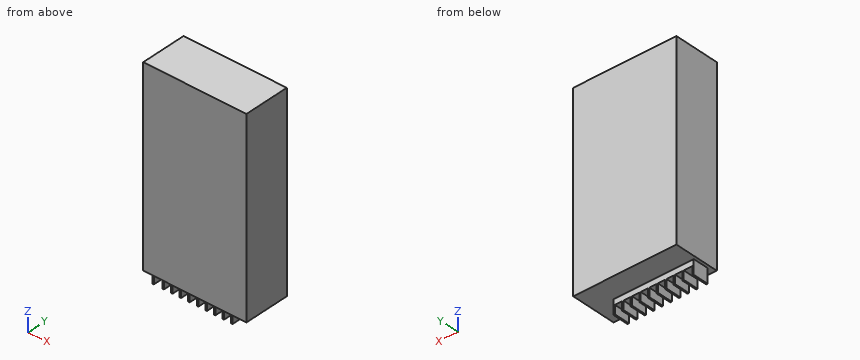
Autodesk Inventor part; units mm, degrees
ref_plane "YZ Plane" through (0, 0, 0) normal (1, 0, 0) x (0, 1, 0)
ref_plane "XZ Plane" through (0, 0, 0) normal (0, 1, 0) x (-1, 0, 0)
ref_plane "XY Plane" through (0, 0, 0) normal (0, 0, 1) x (1, 0, 0)
sketch "Sketch1" plane through (0, 0, 0) normal (0, 0, 1) x (1, 0, 0)
  line L0 (0, 0) -> (114.3, 0)
  line L1 (114.3, 0) -> (114.3, 50.8)
  line L2 (114.3, 50.8) -> (0, 50.8)
  line L3 (0, 50.8) -> (0, 0)
  dimension "d0" = 114.3
  dimension "d1" = 50.8
extrude "Extrusion1" add sketch "Sketch1" against normal blind 211.1375
sketch "Sketch2" plane through (0, 0, -211.1375) normal (0, 0, -1) x (-1, 0, 0)
  line L0 (-114.3, 0) -> (0, 0)
  line L1 (0, 0) -> (0, 50.8)
  line L2 (0, 50.8) -> (-114.3, 50.8)
  line L3 (-114.3, 50.8) -> (-114.3, 0)
  line L4 (-3.175, 7.9375) -> (-92.075, 7.9375)
  line L5 (-92.075, 7.9375) -> (-92.075, 25.4)
  line L6 (-92.075, 25.4) -> (-3.175, 25.4)
  line L7 (-3.175, 25.4) -> (-3.175, 7.9375)
  line L8 (-82.55, 25.4) -> (-80.9625, 25.4)
  line L9 (-80.9625, 25.4) -> (-80.9625, 7.9375)
  line L10 (-80.9625, 7.9375) -> (-82.55, 7.9375)
  line L11 (-82.55, 7.9375) -> (-82.55, 25.4)
  line L12 (-73.025, 25.4) -> (-71.4375, 25.4)
  line L13 (-71.4375, 25.4) -> (-71.4375, 7.9375)
  line L14 (-71.4375, 7.9375) -> (-73.025, 7.9375)
  line L15 (-73.025, 7.9375) -> (-73.025, 25.4)
  line L16 (-63.5, 25.4) -> (-61.9125, 25.4)
  line L17 (-61.9125, 25.4) -> (-61.9125, 7.9375)
  line L18 (-61.9125, 7.9375) -> (-63.5, 7.9375)
  line L19 (-63.5, 7.9375) -> (-63.5, 25.4)
  line L20 (-53.975, 25.4) -> (-52.3875, 25.4)
  line L21 (-52.3875, 25.4) -> (-52.3875, 7.9375)
  line L22 (-52.3875, 7.9375) -> (-53.975, 7.9375)
  line L23 (-53.975, 7.9375) -> (-53.975, 25.4)
  line L24 (-44.45, 25.4) -> (-42.8625, 25.4)
  line L25 (-42.8625, 25.4) -> (-42.8625, 7.9375)
  line L26 (-42.8625, 7.9375) -> (-44.45, 7.9375)
  line L27 (-44.45, 7.9375) -> (-44.45, 25.4)
  line L28 (-34.925, 25.4) -> (-33.3375, 25.4)
  line L29 (-33.3375, 25.4) -> (-33.3375, 7.9375)
  line L30 (-33.3375, 7.9375) -> (-34.925, 7.9375)
  line L31 (-34.925, 7.9375) -> (-34.925, 25.4)
  line L32 (-25.4, 25.4) -> (-23.8125, 25.4)
  line L33 (-23.8125, 25.4) -> (-23.8125, 7.9375)
  line L34 (-23.8125, 7.9375) -> (-25.4, 7.9375)
  line L35 (-25.4, 7.9375) -> (-25.4, 25.4)
  line L36 (-15.875, 25.4) -> (-14.2875, 25.4)
  line L37 (-14.2875, 25.4) -> (-14.2875, 7.9375)
  line L38 (-14.2875, 7.9375) -> (-15.875, 7.9375)
  line L39 (-15.875, 7.9375) -> (-15.875, 25.4)
  line L40 (-4.7625, 25.4) -> (-3.175, 25.4)
  line L41 (-3.175, 25.4) -> (-3.175, 7.9375)
  line L42 (-3.175, 7.9375) -> (-4.7625, 7.9375)
  line L43 (-4.7625, 7.9375) -> (-4.7625, 25.4)
  line L44 (-90.4875, 25.4) -> (-92.075, 25.4)
  line L45 (-92.075, 25.4) -> (-92.075, 7.9375)
  line L46 (-92.075, 7.9375) -> (-90.4875, 7.9375)
  line L47 (-90.4875, 7.9375) -> (-90.4875, 25.4)
  dimension "d4" = 3.175
  dimension "d5" = 7.9375
  dimension "d6" = 22.225
  dimension "d7" = 25.4
  dimension "d8" = 1.5875
  dimension "d9" = 7.9375
  dimension "d10" = 1.5875
  dimension "d11" = 7.9375
  dimension "d12" = 1.5875
  dimension "d13" = 7.9375
  dimension "d14" = 1.5875
  dimension "d15" = 7.9375
  dimension "d16" = 1.5875
  dimension "d17" = 7.9375
  dimension "d18" = 1.5875
  dimension "d19" = 1.5875
  dimension "d21" = 1.5875
  dimension "d23" = 1.5875
  dimension "d24" = 7.9375
  dimension "d25" = 1.5875
  dimension "d26" = 7.9375
  dimension "d27" = 7.9375
extrude "Extrusion2" add sketch "Sketch2" along normal blind 15.875 contours L4 L43 L6 L7 | L4 L39 L6 L37 | L4 L35 L6 L33 | L4 L31 L6 L29 | L4 L27 L6 L25 | L4 L23 L6 L21 | L4 L19 L6 L17 | L4 L15 L6 L13 | L4 L11 L6 L9 | L4 L5 L6 L47
sketch "Sketch3" plane through (0, 0, -211.1375) normal (0, 0, -1) x (-1, 0, 0)
  line L0 (-71.4375, 7.9375) -> (-73.025, 7.9375)
  line L1 (-73.025, 7.9375) -> (-73.025, 25.4)
  line L2 (-52.3875, 7.9375) -> (-53.975, 7.9375)
  line L3 (-53.975, 7.9375) -> (-53.975, 25.4)
  line L4 (-33.3375, 7.9375) -> (-34.925, 7.9375)
  line L5 (-34.925, 7.9375) -> (-34.925, 25.4)
  line L6 (-23.8125, 7.9375) -> (-25.4, 7.9375)
  line L7 (-25.4, 7.9375) -> (-25.4, 25.4)
  line L8 (-14.2875, 7.9375) -> (-15.875, 7.9375)
  line L9 (-15.875, 7.9375) -> (-15.875, 25.4)
  line L10 (-42.8625, 7.9375) -> (-44.45, 7.9375)
  line L11 (-44.45, 7.9375) -> (-44.45, 25.4)
  line L12 (-61.9125, 7.9375) -> (-63.5, 7.9375)
  line L13 (-63.5, 7.9375) -> (-63.5, 25.4)
  line L14 (-80.9625, 7.9375) -> (-82.55, 7.9375)
  line L15 (-82.55, 7.9375) -> (-82.55, 25.4)
  line L16 (-92.075, 25.4) -> (-3.175, 25.4)
  line L17 (-3.175, 25.4) -> (-3.175, 7.9375)
  line L18 (-3.175, 7.9375) -> (-92.075, 7.9375)
  line L19 (-92.075, 7.9375) -> (-92.075, 25.4)
  line L20 (-90.4875, 7.9375) -> (-92.075, 7.9375)
  line L21 (-92.075, 7.9375) -> (-92.075, 25.4)
  line L22 (-92.075, 25.4) -> (-90.4875, 25.4)
  line L23 (-90.4875, 25.4) -> (-90.4875, 7.9375)
  line L24 (-82.55, 25.4) -> (-80.9625, 25.4)
  line L25 (-80.9625, 25.4) -> (-80.9625, 7.9375)
  line L26 (-80.9625, 7.9375) -> (-82.55, 7.9375)
  line L27 (-82.55, 7.9375) -> (-82.55, 25.4)
  line L28 (-73.025, 25.4) -> (-71.4375, 25.4)
  line L29 (-71.4375, 25.4) -> (-71.4375, 7.9375)
  line L30 (-71.4375, 7.9375) -> (-73.025, 7.9375)
  line L31 (-73.025, 7.9375) -> (-73.025, 25.4)
  line L32 (-63.5, 25.4) -> (-61.9125, 25.4)
  line L33 (-61.9125, 25.4) -> (-61.9125, 7.9375)
  line L34 (-61.9125, 7.9375) -> (-63.5, 7.9375)
  line L35 (-63.5, 7.9375) -> (-63.5, 25.4)
  line L36 (-53.975, 25.4) -> (-52.3875, 25.4)
  line L37 (-52.3875, 25.4) -> (-52.3875, 7.9375)
  line L38 (-52.3875, 7.9375) -> (-53.975, 7.9375)
  line L39 (-53.975, 7.9375) -> (-53.975, 25.4)
  line L40 (-44.45, 25.4) -> (-42.8625, 25.4)
  line L41 (-42.8625, 25.4) -> (-42.8625, 7.9375)
  line L42 (-42.8625, 7.9375) -> (-44.45, 7.9375)
  line L43 (-44.45, 7.9375) -> (-44.45, 25.4)
  line L44 (-34.925, 25.4) -> (-33.3375, 25.4)
  line L45 (-33.3375, 25.4) -> (-33.3375, 7.9375)
  line L46 (-33.3375, 7.9375) -> (-34.925, 7.9375)
  line L47 (-34.925, 7.9375) -> (-34.925, 25.4)
  line L48 (-25.4, 25.4) -> (-23.8125, 25.4)
  line L49 (-23.8125, 25.4) -> (-23.8125, 7.9375)
  line L50 (-23.8125, 7.9375) -> (-25.4, 7.9375)
  line L51 (-25.4, 7.9375) -> (-25.4, 25.4)
  line L52 (-15.875, 25.4) -> (-14.2875, 25.4)
  line L53 (-14.2875, 25.4) -> (-14.2875, 7.9375)
  line L54 (-14.2875, 7.9375) -> (-15.875, 7.9375)
  line L55 (-15.875, 7.9375) -> (-15.875, 25.4)
  line L56 (-4.7625, 25.4) -> (-3.175, 25.4)
  line L57 (-3.175, 25.4) -> (-3.175, 7.9375)
  line L58 (-3.175, 7.9375) -> (-4.7625, 7.9375)
  line L59 (-4.7625, 7.9375) -> (-4.7625, 25.4)
extrude "Extrusion3" add sketch "Sketch3" along normal blind 6.35 contours L29 L16 L13 L18 | L18 L25 L16 L1 | L33 L16 L3 L18 | L18 L23 L16 L15 | L37 L16 L11 L18 | L41 L16 L5 L18 | L45 L16 L7 L18 | L49 L16 L9 L18 | L53 L16 L59 L18
properties part number "powerSupply"
Input: part model. Units: mm. Frame: model coordinates. Give positions to 0.01 mm unless a question says otherwise; leave off trailing zeros. Write each loop counter-clockwise with the first axis right and the second up, starting at its lowest first coordinate (ties: lowest second). Pieces come first, ordered by that corner, then holes. Notation, with made-up numbers: M 45,83 L 69,83 A12 cw 69,105 Z; hole C 57.5,68.25 d10. An arc over 180 degrees is marked long. Use one line per item in the form item = value.
1. Cut plane B-B on y = 5.5. Return loops of the section in (x, z), and give its area (3 significant figures).
Outcome:
outline = M 0,-211.14 L 114.3,-211.14 L 114.3,0 L 0,0 Z
area = 24,100 mm²
2. Cut plane A-A on x = 47.5. Return loops of the section in (y, z).
Outcome:
outline = M 0,-211.14 L 7.94,-211.14 L 7.94,-217.49 L 25.4,-217.49 L 25.4,-211.14 L 50.8,-211.14 L 50.8,0 L 0,0 Z
3. Ray query, L1, parallel to Z at x = 82.5, y = 45; L2, parallel to Z at x = 67, y = 21.5. Return the intervals inside material, ascending.
Outcome:
L1 = -211.14 to 0
L2 = -217.49 to 0
4. Cut plane C-C on x = 98.5. Return loops of the section in (y, z), and give its area (3 significant figures).
Outcome:
outline = M 0,-211.14 L 50.8,-211.14 L 50.8,0 L 0,0 Z
area = 10,700 mm²
5. First-contact query: P1, Ø5, axis at y = 19, z = -222, coming from the +X side (3 decimals); P2, Ø8, axis at y = 13.5, z = -220, coming from the -X side (3 decimals); P3, Ø10, axis at y = 31.5, z = -56, coming from the -X side; P4, Ø12.5, axis at x = 42.5, z = -217.5, coming from the +Y side. Flat tips, straight axial feed; report the tip coordinate or a pass-through.
Outcome:
P1 = 92.075
P2 = 3.175
P3 = 0
P4 = 25.4
